from build123d import *

# Parameters (mm, degrees)
BOSS_EXTRUDE2_DEPTH   = 76.2
BOSS_EXTRUDE2_2_DEPTH = 76.2
BOSS_EXTRUDE3_DEPTH   = 12.7
BOSS_EXTRUDE4_DEPTH   = 12.7
SKETCH3_R             = 2.1
CUT_EXTRUDE1_DEPTH    = 6.35


with BuildPart() as part:
    # Sketch1 → Boss-Extrude2 (new body)
    with BuildSketch(Plane(origin=(0, 0, 0), x_dir=(1, 0, 0), z_dir=(0, 1, 0))):
        Polygon((25.4, 0), (0, 0), (0, 25.4), (0, 30.48), (-5.08, 30.48), (-5.08, -5.08), (30.48, -5.08), (30.48, 0), align=None)
    extrude(amount=BOSS_EXTRUDE2_DEPTH)



with BuildPart() as body_2:
    # Sketch1 → Boss-Extrude2 2 (new body)
    with BuildSketch(Plane(origin=(0, 0, 0), x_dir=(1, 0, 0), z_dir=(0, 1, 0))):
        Polygon((8.255, 30.48), (3.175, 30.48), (3.175, 25.4), (3.175, 3.175), (25.4, 3.175), (30.48, 3.175), (30.48, 8.255), (8.255, 8.255), align=None)
    extrude(amount=BOSS_EXTRUDE2_2_DEPTH)


with BuildPart() as part_1:
    add(part.part)

    add(body_2.part)  # Boss-Extrude3 merges body 2
    # Sketch1_5 → Boss-Extrude3 (add)
    with BuildSketch(Plane(origin=(0, 0, 0), x_dir=(1, 0, 0), z_dir=(0, 1, 0))):
        Polygon((0, 25.4), (0, 0), (25.4, 0), (30.48, 0), (30.48, 3.175), (25.4, 3.175), (3.175, 3.175), (3.175, 25.4), (3.175, 30.48), (0, 30.48), align=None)
    extrude(amount=BOSS_EXTRUDE3_DEPTH)

    # Sketch2 → Boss-Extrude4 (add)
    with BuildSketch(Plane(origin=(0, 76.2, 0), x_dir=(1, 0, 0), z_dir=(0, 1, 0))):
        Polygon((8.255, 8.255), (8.255, 30.48), (3.175, 30.48), (3.175, 3.175), (30.48, 3.175), (30.48, 8.255), align=None)
        Polygon((30.48, 0), (30.48, 3.175), (3.175, 3.175), (3.175, 30.48), (0, 30.48), (0, 0), align=None)
        Polygon((30.48, 0), (0, 0), (0, 30.48), (-5.08, 30.48), (-5.08, -5.08), (30.48, -5.08), align=None)
    extrude(amount=-BOSS_EXTRUDE4_DEPTH)

    # Sketch3 → Cut-Extrude1 (cut)
    with BuildSketch(Plane.XZ):
        with Locations(Location((1.5875, -19.3675, 0), (0, 0, 270))):
            Circle(SKETCH3_R)
        with Locations(Location((19.3675, -1.5875, 0), (0, 0, 270))):
            Circle(SKETCH3_R)
    extrude(amount=-CUT_EXTRUDE1_DEPTH, mode=Mode.SUBTRACT)


solid = part_1.part
Source: CAD feature listing. Evaluate the final solid. Frame: model axes, mm. A direction names the side the tool comes from. Coordinates: 2 decimals unless noted, no trailing zeros. Order: outer loops, then holes, each group sorted by start corner. A loop starts at its lowest first (then second) coordinate and runs counter-clockwise, first axis right, second up. Notation, with made-up numbers: M -38,79 L -32,79 A20 ccw -32,115 Z; hole C 53.25,17.5 d9. An arc over 180 degrees is marked long. Write each question's results on one line, items separated by ' | '. Start each with the question number.
1. Reachability of faces 4 (the face through (20, 38, -8.255)), 5 (the face through (8, 12.7, -3)), 6 (the face through (15, 38, 0)) from +Z, -Z, +X, -X, +Y, -Y: full face, straight path, thin tool, end or side. Return the list, or none.
2. Section C-C, the plane x = 23.5. Return the cut outline in (y, z) (3 decimals).
3. Section A-A, the plane y = 31. Return the cut outline in (x, z) (3 decimals), then the cut area to 3 significant figures.
4. Draft query along Y for faces 1 (the face through (30.48, 38, 1)), 2 (the face through (17, 38, -3.175)), 3 (the face through (5, 76.2, -9)). Return one class per face: +Y half, -Y half, draft (parallel to the pull), parting line (faces both ways), or undercut.
5. Section D-D, the plane y = 10. Return the cut outline in (x, z) (3 decimals), then the cut area to 3 significant figures.
6. Material intervals for L1, parallel to X at y = 26, z = -21 (3 decimals); L2, parallel to Z at x = 11.5, y = 15.5 (3 decimals); L3, parallel to Y at x = 0.5, z = -26, sorted ascending.
7. Pin query (flat end, axial travel): pin 1 (4 mm diameter, centred on x = 19.37, z = -1.59, fed in from -Y); pin 2 (18 mm diameter, centred on y = 21.5, z = -23, fed in from +X) (3 decimals); pin 3 (5 mm diameter, centred on x = 12, y = 42.5, fed in from -Z) (3 decimals). Return the tip coordinate at first contact, or that it passes through.
8. Section B-B, the plane z = -11.5. Return the cut outline in (x, y) (3 decimals), then the cut area to 3 significant figures.
Solution:
1) face 4: -Z, +X, +Y, -Y | face 5: none | face 6: +X
2) outline: M 0,-8.255 L 76.2,-8.255 L 76.2,5.08 L 0,5.08 Z; hole M 12.7,-3.175 L 63.5,-3.175 L 63.5,0 L 12.7,0 Z
3) outline: M -5.08,-30.48 L 0,-30.48 L 0,0 L 30.48,0 L 30.48,5.08 L -5.08,5.08 Z; M 3.175,-30.48 L 8.255,-30.48 L 8.255,-8.255 L 30.48,-8.255 L 30.48,-3.175 L 3.175,-3.175 Z | area: 587 mm²
4) face 1: draft | face 2: undercut | face 3: +Y half
5) outline: M -5.08,-30.48 L 8.255,-30.48 L 8.255,-8.255 L 30.48,-8.255 L 30.48,5.08 L -5.08,5.08 Z | area: 771 mm²
6) L1: -5.08 to 0, 3.175 to 8.255 | L2: -8.255 to -3.175, 0 to 5.08 | L3: 0 to 12.7, 63.5 to 76.2
7) pin 1: y = 6.35 | pin 2: x = 8.255 | pin 3: z = -8.255
8) outline: M -5.08,0 L 8.255,0 L 8.255,76.2 L -5.08,76.2 Z; hole M 0,12.7 L 3.175,12.7 L 3.175,63.5 L 0,63.5 Z | area: 855 mm²
